```python
from build123d import *

# Parameters (mm, degrees)
F0_R     = 101
F1_DEPTH = 200
F2_R     = 20
F3_R     = 100
F4_DEPTH = 180
F5_R     = 116
F5_R_2   = 101
F6_DEPTH = 15
F7_R     = 14.99999


# Not quite as in the source:
# - a fillet or chamfer is up to 0.001 mm smaller than in the source, because OpenCascade refuses the exact size


with BuildPart() as f1:
    # F0 (on Top) → F1 (new body)
    with BuildSketch(Plane.XY):
        Circle(F0_R)
    extrude(amount=F1_DEPTH)

    # F2
    f2_edges = [f1.edges().sort_by_distance(p)[0] for p in [
        (-101, 0, 0),
    ]]
    fillet(f2_edges, radius=F2_R)

    # F3 (on face) → F4 (cut)
    with BuildSketch(Plane.XY.offset(200)):
        Circle(F3_R)
    extrude(amount=-F4_DEPTH, mode=Mode.SUBTRACT)

    # F5 (on face) → F6 (join)
    with BuildSketch(Plane.XY.offset(200)):
        Circle(F5_R)
        Circle(F5_R_2, mode=Mode.SUBTRACT)
    extrude(amount=-F6_DEPTH)

    # F7 (radius 15 in the source; OpenCascade refuses exactly that, so slightly less here)
    f7_edges = [f1.edges().sort_by_distance(p)[0] for p in [
        (-116, 0, 200),
    ]]
    fillet(f7_edges, radius=F7_R)


solid = f1.part
```
Read the model definition and answer for the solid it produces. Units are mm, in the model's axes. A direction names the side the tool comes from. Give positions to 0.01 mm unless a question says otherwise; leave off trailing zeros. Write each loop counter-clockwise with the first axis right and the second up, starting at its lowest first coordinate (ties: lowest second). Pieces come first, ordered by that corner, then holes. Notation, with made-up numbers: (-4.75, 0) - (28.25, 0) arc R16 ccw to (28.25, 24) - close; hole circle Ø9 at (77.5, 30). An arc over 180 degrees is marked (long way). Write item = value, one per line. Start each with the question number.
Item 1: Find section C-C (z = 178). Give the vertices of the cut face in (x, y).
Item 2: Each of these flat-tipped pins is pushed along its axis until it touches: P1, Ø10, axis at x = 67, y = -29, coming from the +Z side; P2, Ø10, axis at y = 63, z = 46, coming from the +X side; P3, Ø5, axis at x = 54, z = 40, coming from the +Y side; P4, Ø5, axis at x = -83, y = -87.5, coming from the +Z side. Where does it stop, or does it pass through?
Item 3: A tool of negligible diameter and unlimited length cuts with its end or side. For faces 1 (the flat face through (-1, 1, 0)), 2 (the flat face through (-1, 1, 20)), from which of +Z, -Z, +X, -X, +Y, -Y can it reach the whole face along a straight path? Write none if from no direction.
Item 4: The mould has two halves that part along X. Classify faces 3 (the cylindrical face through (95.38, 30.04, 111.26)), 4 (the flat face through (-35, 95, 185)), 5 (the cylindrical face through (-21.89, -98.6, 101.34)): +X half, -X half, draft (parallel to the pull), parting line (faces both ways), or undercut.
Item 5: Find the intervals of material crossed by probe 1 along Y at (x, z) = (0, 99); probe 2 along Z at (x, y) = (-51, 8); probe 3 along X at (y, z) = (-11, 178.5), in increasing order. Write a range as [from, to].
Response:
q1.outline = circle Ø202 at (0, 0); hole circle Ø200 at (0, 0)
q2.P1 = 20
q2.P2 = 82.69
q2.P3 = 86.88
q2.P4 = through
q3.face_1 = -Z, +X, -X, +Y, -Y
q3.face_2 = +Z
q4.face_3 = undercut
q4.face_4 = draft
q4.face_5 = parting line
q5.probe_1 = [-101, -100], [100, 101]
q5.probe_2 = [0, 20]
q5.probe_3 = [-100.4, -99.39], [99.39, 100.4]
